For this review, take the finished solid that the model builds, in its own axes (mm). Coordinates: 2 decimals unless noted, no trailing zeros. Loops run counter-clockwise (first coordinate to the right, second up) from the corner with the lowest first, then second, coordinate; pieces in that order, holes last. Notation, with made-up numbers: (-37, 24.25) - (-12, 24.25) arc R16 cw to (-12, 39.25) - close; hole circle Ø7 at (74.25, 75). An arc over 180 degrees is marked (long way). Use one line per item in the form item = value. Start each with the question number.
1. For pin 1 Ø10 at (y, z) = (15, -15.5) entering from -X; pin 2 Ø3 at (y, z) = (10, -17.5) entering from -X, all flat-tipped, find the tip position at first contact; note any pin that passes through.
2. Add section A-A on z = -17.5. Give the boundary of the cut face in (x, y), and give its area (3 significant figures).
3. Draft analysis for pull direction Z (two halves, no side actions). For faces 1 (the face through (10, 10, -12)), 2 (the face through (5, 10, -25)), 3 (the face through (4.93, 11.939, -18.736)), 4 (the face through (5.07, 0.9, -0.86)), state which applies: +Z half, -Z half, draft (parallel to the pull), parting line (faces both ways), or undercut.
4. Add section C-C on y = 10. Give the boundary of the cut face in (x, z).
5. To check wall thickness, follow probe 1 along Y at (x, z) = (7, -7.5); probe 2 along Z at (x, y) = (1, 11); probe 3 along Z at (x, y) = (6.75, 8.5). State the ranges of each line that lie inside material, in increasing order.
6. Add section D-D on y = 8. Give the boundary of the cut face in (x, z), and give its area (3 significant figures).
7. Add section B-B on x = 5. Give the boundary of the cut face in (y, z), and give its area (3 significant figures).
```python
from build123d import *

# Parameters (mm, degrees)
SKETCH_1_W      = 25
SKETCH_1_H      = 20
SKETCH_1_R      = 2.3
EXTRUDE_1_DEPTH = 10
FILLET_1_R      = 3


with BuildPart() as part:
    # 草图1 → 凸台-拉伸1 (new body)
    with BuildSketch(Plane(origin=(0, 0, 0), x_dir=(0, 0, -1), z_dir=(1, 0, 0))):
        with Locations((12.5, 10)):
            Rectangle(SKETCH_1_W, SKETCH_1_H)
        with Locations((7.5, 10)):
            Circle(SKETCH_1_R, mode=Mode.SUBTRACT)
        with Locations((17.5, 10)):
            Circle(SKETCH_1_R, mode=Mode.SUBTRACT)
    extrude(amount=EXTRUDE_1_DEPTH)

    # 圆角1
    fillet_1_edges = [part.edges().sort_by_distance(p)[0] for p in [
        (5, 20, 0),
        (5, 20, -25),
        (5, 0, -25),
        (5, 0, 0),
    ]]
    fillet(fillet_1_edges, radius=FILLET_1_R)


solid = part.part
```
Conclusion:
q1.pin_1 = 0
q1.pin_2 = through
q2.outline = (0, 0) - (10, 0) - (10, 7.7) - (0, 7.7) - close; (0, 12.3) - (10, 12.3) - (10, 20) - (0, 20) - close
q2.area = 154 mm^2
q3.face_1 = draft
q3.face_2 = -Z half
q3.face_3 = undercut
q3.face_4 = +Z half
q4.outline = (0, -25) - (10, -25) - (10, -19.8) - (0, -19.8) - close; (0, -15.2) - (10, -15.2) - (10, -9.8) - (0, -9.8) - close; (0, -5.2) - (10, -5.2) - (10, 0) - (0, 0) - close
q5.probe_1 = 0 to 7.7, 12.3 to 20
q5.probe_2 = -25 to -19.57, -15.43 to -9.57, -5.43 to 0
q5.probe_3 = -25 to -19.24, -15.76 to -9.24, -5.76 to 0
q6.outline = (0, -25) - (10, -25) - (10, -18.64) - (0, -18.64) - close; (0, -16.36) - (10, -16.36) - (10, -8.64) - (0, -8.64) - close; (0, -6.36) - (10, -6.36) - (10, 0) - (0, 0) - close
q6.area = 205 mm^2
q7.outline = (0, -22) arc R3 ccw to (3, -25) - (17, -25) arc R3 ccw to (20, -22) - (20, -3) arc R3 ccw to (17, 0) - (3, 0) arc R3 ccw to (0, -3) - close; hole circle Ø4.6 at (10, -17.5); hole circle Ø4.6 at (10, -7.5)
q7.area = 459 mm^2
